```python
from build123d import *

# Parameters (mm, degrees)
SKETCH1_W           = 100
SKETCH1_H           = 100
BOSS_EXTRUDE1_DEPTH = 12
CUT_EXTRUDE1_REACH  = 88.856
SKETCH2_R           = 3
CUT_EXTRUDE2_REACH  = 88.856
SKETCH3_R           = 2
SKETCH3_R_2         = 13
CUT_EXTRUDE3_REACH  = 88.856
SKETCH4_R           = 6


with BuildPart() as part:
    # Sketch1 → Boss-Extrude1 (new body)
    with BuildSketch(Plane(origin=(0, 0, 0), x_dir=(1, 0, 0), z_dir=(0, 1, 0))):
        with Locations((0, -20)):
            Rectangle(SKETCH1_W, SKETCH1_H)
    extrude(amount=BOSS_EXTRUDE1_DEPTH)

    # Sketch2 → Cut-Extrude1 (cut, up to next)
    with BuildSketch(Plane(origin=(0, 12, 0), x_dir=(1, 0, 0), z_dir=(0, 1, 0)), mode=Mode.PRIVATE) as cut_extrude1_sk1:
        with Locations(Location((-44, 20, 0), (0, 0, 270))):
            Circle(SKETCH2_R)
    cut_extrude1_tool1 = extrude(cut_extrude1_sk1.sketch, amount=-CUT_EXTRUDE1_REACH, mode=Mode.PRIVATE) & part.part
    # Sketch2 → Cut-Extrude1 (cut, up to next)
    with BuildSketch(Plane(origin=(0, 12, 0), x_dir=(1, 0, 0), z_dir=(0, 1, 0)), mode=Mode.PRIVATE) as cut_extrude1_sk2:
        with Locations(Location((-44, 0, 0), (0, 0, 270))):
            Circle(SKETCH2_R)
    cut_extrude1_tool2 = extrude(cut_extrude1_sk2.sketch, amount=-CUT_EXTRUDE1_REACH, mode=Mode.PRIVATE) & part.part
    # Sketch2 → Cut-Extrude1 (cut, up to next)
    with BuildSketch(Plane(origin=(0, 12, 0), x_dir=(1, 0, 0), z_dir=(0, 1, 0)), mode=Mode.PRIVATE) as cut_extrude1_sk3:
        with Locations(Location((44, 20, 0), (0, 0, 270))):
            Circle(SKETCH2_R)
    cut_extrude1_tool3 = extrude(cut_extrude1_sk3.sketch, amount=-CUT_EXTRUDE1_REACH, mode=Mode.PRIVATE) & part.part
    # Sketch2 → Cut-Extrude1 (cut, up to next)
    with BuildSketch(Plane(origin=(0, 12, 0), x_dir=(1, 0, 0), z_dir=(0, 1, 0)), mode=Mode.PRIVATE) as cut_extrude1_sk4:
        with Locations(Location((44, 0, 0), (0, 0, 270))):
            Circle(SKETCH2_R)
    cut_extrude1_tool4 = extrude(cut_extrude1_sk4.sketch, amount=-CUT_EXTRUDE1_REACH, mode=Mode.PRIVATE) & part.part
    add(cut_extrude1_tool1.solids().sort_by_distance((-44, 12, -20))[0], mode=Mode.SUBTRACT)
    add(cut_extrude1_tool2.solids().sort_by_distance((-44, 12, 0))[0], mode=Mode.SUBTRACT)
    add(cut_extrude1_tool3.solids().sort_by_distance((44, 12, -20))[0], mode=Mode.SUBTRACT)
    add(cut_extrude1_tool4.solids().sort_by_distance((44, 12, 0))[0], mode=Mode.SUBTRACT)

    # Sketch3 → Cut-Extrude2 (cut, up to next)
    with BuildSketch(Plane(origin=(0, 12, 0), x_dir=(1, 0, 0), z_dir=(0, 1, 0)), mode=Mode.PRIVATE) as cut_extrude2_sk1:
        with Locations(Location((-23.5, -43.5, 0), (0, 0, 270))):
            Circle(SKETCH3_R)
    cut_extrude2_tool1 = extrude(cut_extrude2_sk1.sketch, amount=-CUT_EXTRUDE2_REACH, mode=Mode.PRIVATE) & part.part
    # Sketch3 → Cut-Extrude2 (cut, up to next)
    with BuildSketch(Plane(origin=(0, 12, 0), x_dir=(1, 0, 0), z_dir=(0, 1, 0)), mode=Mode.PRIVATE) as cut_extrude2_sk2:
        with Locations(Location((23.5, -43.5, 0), (0, 0, 270))):
            Circle(SKETCH3_R)
    cut_extrude2_tool2 = extrude(cut_extrude2_sk2.sketch, amount=-CUT_EXTRUDE2_REACH, mode=Mode.PRIVATE) & part.part
    # Sketch3 → Cut-Extrude2 (cut, up to next)
    with BuildSketch(Plane(origin=(0, 12, 0), x_dir=(1, 0, 0), z_dir=(0, 1, 0)), mode=Mode.PRIVATE) as cut_extrude2_sk3:
        with Locations(Location((23.5, 3.5, 0), (0, 0, 270))):
            Circle(SKETCH3_R)
    cut_extrude2_tool3 = extrude(cut_extrude2_sk3.sketch, amount=-CUT_EXTRUDE2_REACH, mode=Mode.PRIVATE) & part.part
    # Sketch3 → Cut-Extrude2 (cut, up to next)
    with BuildSketch(Plane(origin=(0, 12, 0), x_dir=(1, 0, 0), z_dir=(0, 1, 0)), mode=Mode.PRIVATE) as cut_extrude2_sk4:
        with Locations(Location((-23.5, 3.5, 0), (0, 0, 270))):
            Circle(SKETCH3_R)
    cut_extrude2_tool4 = extrude(cut_extrude2_sk4.sketch, amount=-CUT_EXTRUDE2_REACH, mode=Mode.PRIVATE) & part.part
    # Sketch3 → Cut-Extrude2 (cut, up to next)
    with BuildSketch(Plane(origin=(0, 12, 0), x_dir=(1, 0, 0), z_dir=(0, 1, 0)), mode=Mode.PRIVATE) as cut_extrude2_sk5:
        with Locations(Location((0, -20, 0), (0, 0, 270))):
            Circle(SKETCH3_R_2)
    cut_extrude2_tool5 = extrude(cut_extrude2_sk5.sketch, amount=-CUT_EXTRUDE2_REACH, mode=Mode.PRIVATE) & part.part
    add(cut_extrude2_tool1.solids().sort_by_distance((-23.5, 12, 43.5))[0], mode=Mode.SUBTRACT)
    add(cut_extrude2_tool2.solids().sort_by_distance((23.5, 12, 43.5))[0], mode=Mode.SUBTRACT)
    add(cut_extrude2_tool3.solids().sort_by_distance((23.5, 12, -3.5))[0], mode=Mode.SUBTRACT)
    add(cut_extrude2_tool4.solids().sort_by_distance((-23.5, 12, -3.5))[0], mode=Mode.SUBTRACT)
    add(cut_extrude2_tool5.solids().sort_by_distance((0, 12, 20))[0], mode=Mode.SUBTRACT)

    # Sketch4 → Cut-Extrude3 (cut, up to next)
    with BuildSketch(Plane(origin=(0, 12, 0), x_dir=(1, 0, 0), z_dir=(0, 1, 0)), mode=Mode.PRIVATE) as cut_extrude3_sk1:
        with Locations(Location((-36, -40, 0), (0, 0, 270))):
            Circle(SKETCH4_R)
    cut_extrude3_tool1 = extrude(cut_extrude3_sk1.sketch, amount=-CUT_EXTRUDE3_REACH, mode=Mode.PRIVATE) & part.part
    # Sketch4 → Cut-Extrude3 (cut, up to next)
    with BuildSketch(Plane(origin=(0, 12, 0), x_dir=(1, 0, 0), z_dir=(0, 1, 0)), mode=Mode.PRIVATE) as cut_extrude3_sk2:
        with Locations(Location((36, -40, 0), (0, 0, 270))):
            Circle(SKETCH4_R)
    cut_extrude3_tool2 = extrude(cut_extrude3_sk2.sketch, amount=-CUT_EXTRUDE3_REACH, mode=Mode.PRIVATE) & part.part
    add(cut_extrude3_tool1.solids().sort_by_distance((-36, 12, 40))[0], mode=Mode.SUBTRACT)
    add(cut_extrude3_tool2.solids().sort_by_distance((36, 12, 40))[0], mode=Mode.SUBTRACT)


solid = part.part
```
Work out the finished part from the listing and answer in its coordinate system (mm). Give positions to 0.01 mm unless a question says otherwise; leave off trailing zeros. Loops run counter-clockwise (first coordinate to the right, second up) from the corner with the lowest first, then second, coordinate; pieces in that order, holes last. Notation, with made-up numbers: (-14.5, -7) -> (34.5, -7) arc R9 ccw to (34.5, 8) -> close; hole circle Ø10 at (54.25, 21.5). An arc over 180 degrees is marked (long way). Put each result on its own line as item: value. Start each with the question number.
Item 1: The part is cut by section A-A (z = 40). Give the vertices of the cut face in (x, y).
Item 2: Find the intervals of material crossed by L1, parallel to X at y = 3.25, z = -20; L2, parallel to X at y = 6.5, z = 20; L3, parallel to X at y = 8.75, z = 35, in increasing order. Write a range as [from, to].
Item 3: The part is cut by section B-B (x = 23.5). Give the vertices of the cut face in (y, z).
Item 4: This flat-tipped pin is pushed along its axis until it touches: P1, Ø19, axis at x = -36, z = 40, coming from the +Y side. Where does it stop, or does it pass through?
Item 5: The mould has two halves that part along Z. Classify faces 1 (the face through (-39.65, 6.08, 35.24)), 2 (the face through (-1, 6, 70)), 3 (the face through (22.3, 6.1, 41.9)), 4 (the face through (-12, 12, 8)): released by +Z, released by -Z, zero draft, split by the parting line, or undercut.
Item 6: The part is cut by section C-C (z = 20). Give the vertices of the cut face in (x, y), then the cut area to 3 significant figures.
Item 7: The part is cut by section D-D (y = 2.25). State how many separate pieces and enclosed holes the cut face has, then the cut area to 3 significant figures.
Answers below:
1. outline: (-50, 0) -> (-42, 0) -> (-42, 12) -> (-50, 12) -> close; (-30, 0) -> (30, 0) -> (30, 12) -> (-30, 12) -> close; (42, 0) -> (50, 0) -> (50, 12) -> (42, 12) -> close
2. L1: [-50, -47], [-41, 41], [47, 50]
2. L2: [-50, -13], [13, 50]
2. L3: [-50, -39.32], [-32.68, 32.68], [39.32, 50]
3. outline: (0, -30) -> (12, -30) -> (12, -5.5) -> (0, -5.5) -> close; (0, -1.5) -> (12, -1.5) -> (12, 41.5) -> (0, 41.5) -> close; (0, 45.5) -> (12, 45.5) -> (12, 70) -> (0, 70) -> close
4. P1: y = 12
5. face 1: undercut
5. face 2: released by +Z
5. face 3: undercut
5. face 4: zero draft
6. outline: (-50, 0) -> (-13, 0) -> (-13, 12) -> (-50, 12) -> close; (13, 0) -> (50, 0) -> (50, 12) -> (13, 12) -> close
6. area: 888 mm2
7. separate pieces: 1
7. enclosed holes: 11
7. area: 9,080 mm2
